The model under review builds one solid part; all positions refer to its coordinate system, in mm. A direction names the side the tool comes from. Coordinates: 2 decimals unless noted, no trailing zeros. Write each loop counter-clockwise with the first axis right and the second up, starting at its lowest first coordinate (ties: lowest second). Pieces come first, ordered by that corner, then holes. Notation, with made-up numbers: (12.5, -22) - (45.5, -22) arc R29 ccw to (45.5, 4) - close; hole circle Ø10 at (32, -1). An arc over 180 degrees is marked (long way). Return JSON: item names as keys, results as strings. Group by question number.
(1) Tool access review of faces 5 (the face through (0, -9.786, 0)), 6 (the face through (-16, 1, 0)), 7 (the face through (12, -10.786, 0)), 8 (the face through (16, 1, 0)), 9 (the face through (-7.493, 0.33, 13.479)): name each direction out of +Z, -Z, +X, -X, +Y, -Y from which nothing blocks a thin tool from reaching the whole face with its end or side.
(2) We need section C-C on y = -8.25. State the section outline as (x, z) points, then the cut area to 3 significant figures.
(3) We need section D-D on z = -9. State the section outline as (x, y) points, then the cut area to 3 significant figures.
(4) To check wall thickness, follow L1, parallel to Z at x = 12, y = -5.5; L2, parallel to Y at x = 0, z = 13.5; L3, parallel to X at y = 4.5, z = 14. State the ranges of each line that lie inside material, in increasing order. Write a range as from..to.
(5) We need section B-B on z = -0.5. State the section outline as (x, y) points.
(6) For pin 1 Ø5 at (x, z) = (12, -9) entering from +Y; pin 2 Ø1.5 at (x, z) = (2, 10.5) entering from -Y; pin 3 Ø3 at (y, z) = (1.5, -1.5) entering from -X, all flat-tipped, find the tip position at first contact; note any pin that passes through.
(7) We need section A-A on x = 0. State the section outline as (y, z) points.
(8) Draft analysis for pull direction Z (two halves, no side actions). For faces 1 (the face through (-13.474, -2.405, -7.648)), 2 (the face through (-13.474, -2.405, 10.352)), 3 (the face through (4, -7, -15)), 4 (the face through (3, -3, 12)), state which applies: released by +Z, released by -Z, zero draft, split by the parting line, or undercut.
```python
from build123d import *

# Parameters (mm, degrees)
BOSS_EXTRUDE1_DEPTH      = 15
BOSS_EXTRUDE1_DEPTH_BACK = 15
CUT_EXTRUDE1_START       = -12
SKETCH2_R                = 7.5
CUT_EXTRUDE1_DEPTH       = 4
SKETCH3_R                = 4
CUT_EXTRUDE2_DEPTH       = 28
SKETCH4_R                = 2
CUT_EXTRUDE3_DEPTH       = 23


with BuildPart() as part:
    # Sketch1 → Boss-Extrude1 (new body, two sides)
    with BuildSketch(Plane.XY) as boss_extrude1_sk:
        Polygon((17, -10.786397104), (17, -4.786397104), (16, -3.786397104), (16, 6.213602896), (9, 6.213602896), (4, 11.213602896), (-4, 11.213602896), (-9, 6.213602896), (-16, 6.213602896), (-16, -3.786397104), (-17, -4.786397104), (-17, -10.786397104), (-7, -10.786397104), (-6, -9.786397104), (6, -9.786397104), (7, -10.786397104), align=None)
    extrude(amount=BOSS_EXTRUDE1_DEPTH)
    extrude(boss_extrude1_sk.sketch, amount=-BOSS_EXTRUDE1_DEPTH_BACK)

    # Sketch2 → Cut-Extrude1 (cut, through all)
    with BuildSketch(Plane.XY.offset(CUT_EXTRUDE1_START)):
        Circle(SKETCH2_R)
    cut_extrude1 = extrude(amount=-CUT_EXTRUDE1_DEPTH, mode=Mode.SUBTRACT)

    # Mirror1: Cut-Extrude1 across plane
    add(cut_extrude1.mirror(Plane.XY), mode=Mode.SUBTRACT)

    # Sketch3 → Cut-Extrude2 (cut, through all)
    with BuildSketch(Plane.XY.offset(12)):
        Circle(SKETCH3_R)
    extrude(amount=-CUT_EXTRUDE2_DEPTH, mode=Mode.SUBTRACT)

    # Sketch4 → Cut-Extrude3 (cut, through all)
    with BuildSketch(Plane.XZ.offset(10.786397104)):
        with Locations((12, 9)):
            Circle(SKETCH4_R)
        with Locations((-12, 9)):
            Circle(SKETCH4_R)
        with Locations((12, -9)):
            Circle(SKETCH4_R)
        with Locations((-12, -9)):
            Circle(SKETCH4_R)
    extrude(amount=-CUT_EXTRUDE3_DEPTH, mode=Mode.SUBTRACT)


solid = part.part
```
Ans:
{
 "1": {"face 5": "+Z, -Z, -Y", "face 6": "+Z, -Z, -X, +Y", "face 7": "+Z, -Z, +X, -X, -Y", "face 8": "+Z, -Z, +X, +Y", "face 9": "+Z"},
 "2": {"outline": "(-17, -15) - (17, -15) - (17, 15) - (-17, 15) - close; hole circle Ø4 at (-12, -9); hole circle Ø4 at (-12, 9); hole circle Ø4 at (12, -9); hole circle Ø4 at (12, 9)", "area": "970 mm²"},
 "3": {"outline": "(-17, -10.79) - (-14, -10.79) - (-14, 6.21) - (-16, 6.21) - (-16, -3.79) - (-17, -4.79) - close; (-10, -10.79) - (-7, -10.79) - (-6, -9.79) - (6, -9.79) - (7, -10.79) - (10, -10.79) - (10, 6.21) - (9, 6.21) - (4, 11.21) - (-4, 11.21) - (-9, 6.21) - (-10, 6.21) - close; (14, -10.79) - (17, -10.79) - (17, -4.79) - (16, -3.79) - (16, 6.21) - (14, 6.21) - close; hole circle Ø8 at (0, 0)", "area": "423 mm²"},
 "4": {"L1": "-15..-11, -7..7, 11..15", "L2": "-9.79..-7.5, 7.5..11.21", "L3": "-16..-6, 6..16"},
 "5": {"outline": "(-17, -10.79) - (-7, -10.79) - (-6, -9.79) - (6, -9.79) - (7, -10.79) - (17, -10.79) - (17, -4.79) - (16, -3.79) - (16, 6.21) - (9, 6.21) - (4, 11.21) - (-4, 11.21) - (-9, 6.21) - (-16, 6.21) - (-16, -3.79) - (-17, -4.79) - close; hole circle Ø8 at (0, 0)"},
 "6": {"pin 1": "y = 6.21", "pin 2": "y = -9.79", "pin 3": "x = -16"},
 "7": {"outline": "(-9.79, -15) - (-7.5, -15) - (-7.5, -12) - (-4, -12) - (-4, 12) - (-7.5, 12) - (-7.5, 15) - (-9.79, 15) - close; (4, -12) - (7.5, -12) - (7.5, -15) - (11.21, -15) - (11.21, 15) - (7.5, 15) - (7.5, 12) - (4, 12) - close"},
 "8": {"face 1": "undercut", "face 2": "undercut", "face 3": "released by -Z", "face 4": "released by +Z"}
}
